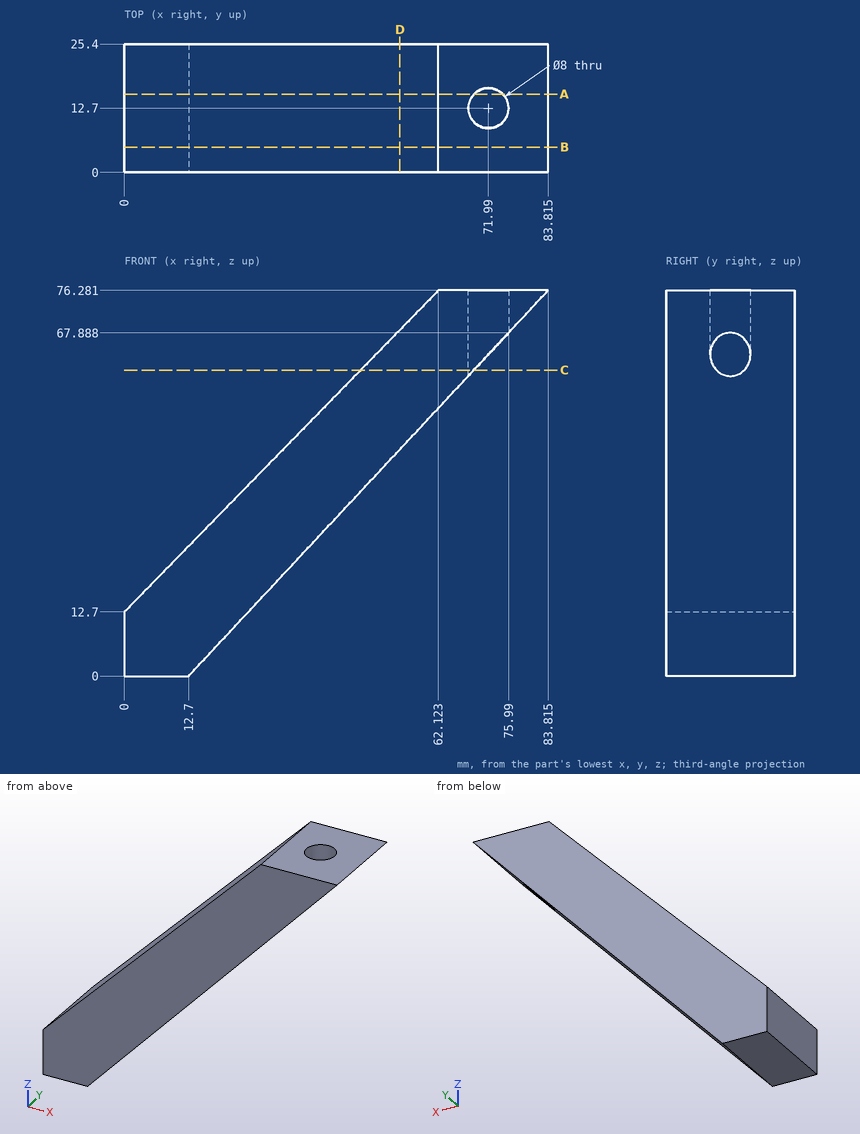
Geometry: see drawing. Coordinates: mm, zero at the bounding-box minimum. Give positions to 0.01 mm unless a question says otherwise; leave off trailing zeros. Write each loop counter-clockwise with the first axis right and the second up, starting at its lowest first coordinate (ties: lowest second). Pieces come first, ordered by that corner, then holes. Notation, with made-up numbers: (-10, -19.75) - (24, -19.75) arc R25 ccw to (24, 5.25) - close; hole circle Ø4 at (78.25, 9.25). An arc over 180 degrees is marked (long way). Return JSON: item names as keys, results as strings. Group by question number.
1) Section D-D on x = 54.5. Return the cut outline in (y, z).
2) Line query: line 1 (X direction, y = 12.7, z = 69) (1 decimal); line 2 (X direction, y = 12.7, z = 71) (1 decimal); line 3 (Z direction, x = 71, y = 3.5) (1 decimal). Output: solid intervals per line, ascending.
3) Section C-C on z = 60.5. Return the cut outline in (x, y) (1 decimal), plus the area to 3 significant figures.
4) Section A-A on y = 15.5. Return the cut outline in (x, z) (1 decimal).
5) Section B-B on y = 5. Return the cut outline in (x, z) (1 decimal).
6) First-contact query: P1, Ø1.5, axis at x = 44.5, y = 20.5, coming from the -Z side (1 decimal); P2, Ø10, axis at x = 24.5, y = 6.5, coming from the -Z side (1 decimal); P3, Ø4, axis at y = 11, z = 39.5, coming from the -X side. Flat tips, straight axial feed; report the tip coordinate or a pass-through.
Filled in:
{
 "1": {"outline": "(0, 44.84) - (25.4, 44.84) - (25.4, 68.48) - (0, 68.48) - close"},
 "2": {"line 1": "x = 55 to 68, 76 to 77", "line 2": "x = 57 to 68, 76 to 78.9", "line 3": "z = 62.5 to 76.3"},
 "3": {"outline": "(46.7, 0) - (69.1, 0) - (69.1, 9.9) arc R4 cw to (69.1, 15.5) - (69.1, 25.4) - (46.7, 25.4) - close", "area": "565 mm^2"},
 "4": {"outline": "(0, 0) - (12.7, 0) - (69.1, 60.5) - (69.1, 76.3) - (62.1, 76.3) - (0, 12.7) - close; (74.8, 66.7) - (83.8, 76.3) - (74.8, 76.3) - close"},
 "5": {"outline": "(0, 0) - (12.7, 0) - (83.8, 76.3) - (62.1, 76.3) - (0, 12.7) - close"},
 "6": {"P1": "stops at z = 33.3", "P2": "stops at z = 7.3", "P3": "stops at x = 24.23"}
}
